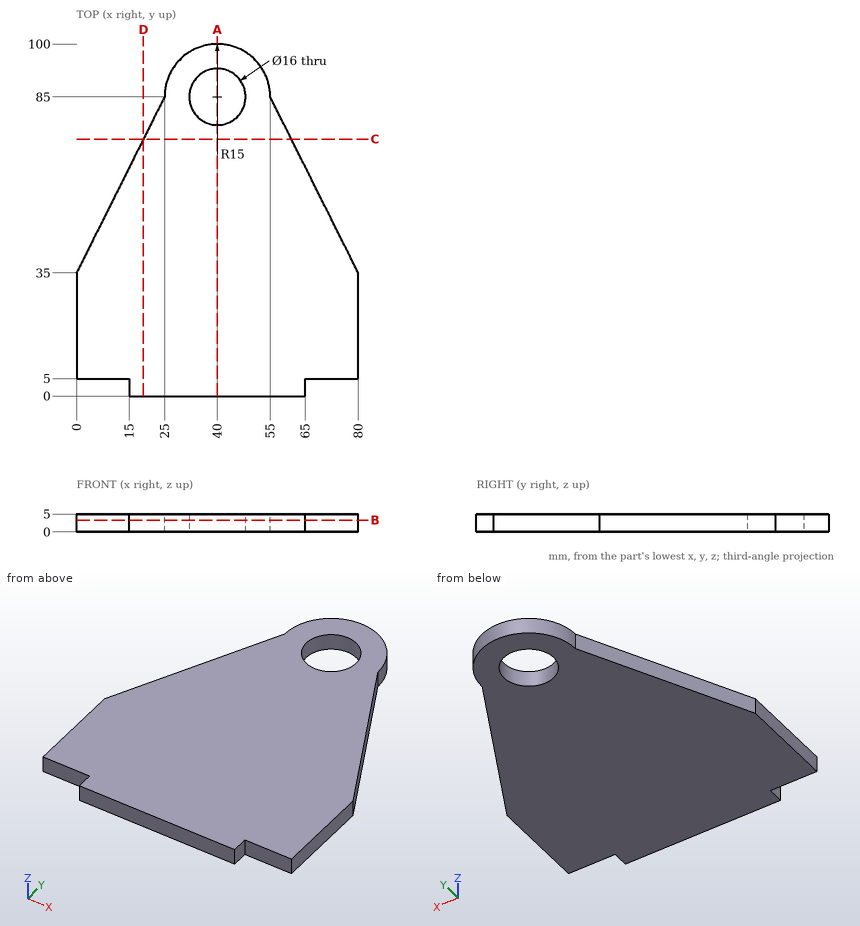
The drawing under review shows one solid part. Ordinate dimensions are in mm from its lowest x, y, z. Give positions to 0.01 mm unless a question says otherwise; leave off trailing zeros. Order: outer loops, then holes, each group sorted by start corner. A loop starts at its lowest first (then second) coordinate and runs counter-clockwise, first axis right, second up. Notation, with made-up numbers: (-29, 61) - (-13, 61) arc R27 ccw to (-13, 77) - close; hole circle Ø11 at (57, -32.75). An arc over 180 degrees is marked (long way). Answer as a JSON object with one key per item and string values. Group by question number.
Item 1: Take a section at B-B on z = 3.3. Give the boundary of the cut face in (x, y), and give its area (3 significant figures).
Item 2: Wall thickness on line 1 along Y through (x, z) = (40, 2.05); line 2 along X through (y, z) = (83, 0.3); line 3 along X through (y, z) = (81, 4.2): over which ranges is each line inside the solid? List them lowest first.
Item 3: Take a section at D-D on x = 19. Give the boundary of the cut face in (y, z), and give its area (3 significant figures).
Item 4: Clearance check with flat-ended pins moving along their axes: pin 1 Ø1.5 at (y, z) = (74.5, 1.5) entering from -X (3 decimals); pin 2 Ø1.5 at (y, z) = (2, 2) entering from +X; pin 3 Ø1.5 at (y, z) = (2, 2) entering from -X. State where each tip first meets the part, or that it passes through.
Item 5: Take a section at C-C on y = 73. Give the boundary of the cut face in (x, z).
Item 6: Take a section at A-A on x = 40. Give the boundary of the cut face in (y, z).
Reported:
{
 "1": {"outline": "(0, 5) - (15, 5) - (15, 0) - (65, 0) - (65, 5) - (80, 5) - (80, 35) - (55, 85) arc R15 ccw to (25, 85) - (0, 35) - close; hole circle Ø16 at (40, 85)", "area": "5,550 mm^2"},
 "2": {"line 1": "0 to 77, 93 to 100", "line 2": "24 to 32.25, 47.75 to 56", "line 3": "23 to 33.07, 46.93 to 57"},
 "3": {"outline": "(0, 0) - (73, 0) - (73, 5) - (0, 5) - close", "area": "365 mm^2"},
 "4": {"pin 1": "x = 19.375", "pin 2": "x = 65", "pin 3": "x = 15"},
 "5": {"outline": "(19, 0) - (61, 0) - (61, 5) - (19, 5) - close"},
 "6": {"outline": "(0, 0) - (77, 0) - (77, 5) - (0, 5) - close; (93, 0) - (100, 0) - (100, 5) - (93, 5) - close"}
}
